The listing builds one solid part. Answer for the finished solid, in the listing's coordinates (mm). A direction names the side the tool comes from. Coordinates: 2 decimals unless noted, no trailing zeros. Order: outer loops, then holes, each group sorted by start corner. A loop starts at its lowest first (then second) coordinate and runs counter-clockwise, first axis right, second up. Notation, with made-up numbers: (85.5, -20) - (105.5, -20) arc R18 ccw to (105.5, -14) - close; hole circle Ø11 at (-18, 3). An arc over 180 degrees is marked (long way). One line per item, written item: value. Start each with the question number.
```python
from build123d import *

# Parameters (mm, degrees)
BOSS_EXTRUDE1_DEPTH = 6
SKETCH2_W           = 20
SKETCH2_H           = 30
BOSS_EXTRUDE2_DEPTH = 4
SKETCH3_W           = 20
SKETCH3_H           = 2
CUT_EXTRUDE1_DEPTH  = 6
SKETCH4_R           = 0.75
CUT_EXTRUDE2_DEPTH  = 172.161563774
SKETCH5_R           = 0.75
CUT_EXTRUDE3_DEPTH  = 153.773797585
SKETCH6_R           = 0.75
CUT_EXTRUDE4_DEPTH  = 174.032600725
SKETCH7_R           = 0.75
CUT_EXTRUDE5_DEPTH  = 191.462831696
FILLET1_R           = 4
SKETCH8_W           = 15
SKETCH8_H           = 30
BOSS_EXTRUDE3_DEPTH = 2
FILLET2_R           = 3
FILLET3_START       = 4.0000001
FILLET3_DEPTH       = 1.9999999
FILLET3_START_2     = 148.554137986
FILLET3_2_DEPTH     = 3.0000001
FILLET3_START_3     = 0.9999999
FILLET3_3_DEPTH     = 3.00000019
SKETCH9_R           = 0.75
CUT_EXTRUDE6_DEPTH  = 12
SKETCH10_R          = 1.1
CUT_EXTRUDE7_DEPTH  = 12
SKETCH11_R          = 1.1
CUT_EXTRUDE8_DEPTH  = 12
SKETCH12_R          = 0.75
CUT_EXTRUDE9_DEPTH  = 12
SKETCH13_R          = 2.1
CUT_EXTRUDE10_DEPTH = 6
SKETCH14_R          = 2.1
CUT_EXTRUDE11_DEPTH = 6


with BuildPart() as part:
    # Sketch1 → Boss-Extrude1 (new body)
    with BuildSketch(Plane.XY):
        Polygon((166.554138086, -30.981559499), (166.554138086, -0.981559499), (102.554138086, -0.981559499), (50.592613859, -30.981559499), (-9.407386141, -30.981559499), (-51.833793012, 11.444847372), (-101.833793012, 11.444847372), (-101.833793012, 7.444847372), (-53.490647262, 7.444847372), (-11.06424039, -34.981559499), (51.664410629, -34.981559499), (103.625934856, -4.981559499), (162.554138086, -4.981559499), (162.554138086, -30.981559499), align=None)
    extrude(amount=BOSS_EXTRUDE1_DEPTH)

    # Sketch2 → Boss-Extrude2 (add)
    with BuildSketch(Plane(origin=(166.554138086, 0, 0), x_dir=(0, 0, -1), z_dir=(1, 0, 0))):
        with Locations((10, -15.981559499)):
            Rectangle(SKETCH2_W, SKETCH2_H)
    extrude(amount=-BOSS_EXTRUDE2_DEPTH)

    # Sketch3 → Cut-Extrude1 (cut)
    with BuildSketch(Plane.XY.offset(6)):
        with Locations((-91.833793012, 8.444847372)):
            Rectangle(SKETCH3_W, SKETCH3_H)
    extrude(amount=-CUT_EXTRUDE1_DEPTH, mode=Mode.SUBTRACT)

    # Sketch4 → Cut-Extrude2 (cut, through all)
    with BuildSketch(Plane(origin=(0, -0.981559499, 0), x_dir=(1, 0, 0), z_dir=(0, 1, 0))):
        with Locations(Location((107.554138086, -3, 0), (0, 0, 180))):
            Circle(SKETCH4_R)
        with Locations(Location((117.554138086, -3, 0), (0, 0, 180))):
            Circle(SKETCH4_R)
        with Locations(Location((127.554138086, -3, 0), (0, 0, 180))):
            Circle(SKETCH4_R)
        with Locations(Location((137.554138086, -3, 0), (0, 0, 180))):
            Circle(SKETCH4_R)
        with Locations(Location((147.554138086, -3, 0), (0, 0, 180))):
            Circle(SKETCH4_R)
        with Locations(Location((157.554138086, -3, 0), (0, 0, 180))):
            Circle(SKETCH4_R)
    extrude(amount=-CUT_EXTRUDE2_DEPTH, mode=Mode.SUBTRACT)

    # Sketch5 → Cut-Extrude3 (cut, through all)
    with BuildSketch(Plane(origin=(26.063562252, -45.143414047, 0), x_dir=(0.8660254037844379, 0.5000000000000013, 0), z_dir=(-0.5000000000000013, 0.8660254037844379, 0))):
        with Locations(Location((33.323709096, -3, 0), (0, 0, 180))):
            Circle(SKETCH5_R)
        with Locations(Location((43.323709096, -3, 0), (0, 0, 180))):
            Circle(SKETCH5_R)
        with Locations(Location((53.323709096, -3, 0), (0, 0, 180))):
            Circle(SKETCH5_R)
        with Locations(Location((63.323709096, -3, 0), (0, 0, 180))):
            Circle(SKETCH5_R)
        with Locations(Location((73.323709096, -3, 0), (0, 0, 180))):
            Circle(SKETCH5_R)
        with Locations(Location((83.323709096, -3, 0), (0, 0, 180))):
            Circle(SKETCH5_R)
    extrude(amount=-CUT_EXTRUDE3_DEPTH, mode=Mode.SUBTRACT)

    # Sketch6 → Cut-Extrude4 (cut, through all)
    with BuildSketch(Plane(origin=(0, -30.981559499, 0), x_dir=(1, 0, 0), z_dir=(0, 1, 0))):
        with Locations(Location((45.592613859, -3, 0), (0, 0, 180))):
            Circle(SKETCH6_R)
        with Locations(Location((35.592613859, -3, 0), (0, 0, 180))):
            Circle(SKETCH6_R)
        with Locations(Location((25.592613859, -3, 0), (0, 0, 180))):
            Circle(SKETCH6_R)
        with Locations(Location((15.592613859, -3, 0), (0, 0, 180))):
            Circle(SKETCH6_R)
        with Locations(Location((5.592613859, -3, 0), (0, 0, 180))):
            Circle(SKETCH6_R)
        with Locations(Location((-4.407386141, -3, 0), (0, 0, 180))):
            Circle(SKETCH6_R)
    extrude(amount=-CUT_EXTRUDE4_DEPTH, mode=Mode.SUBTRACT)

    # Sketch7 → Cut-Extrude5 (cut, through all)
    with BuildSketch(Plane(origin=(-20.19447282, -20.19447282, 0), x_dir=(0, 0, -1), z_dir=(0.7071067811865487, 0.7071067811865464, 0))):
        with Locations(Location((-3, -10.25524428, 0), (0, 0, 90))):
            Circle(SKETCH7_R)
        with Locations(Location((-3, -0.25524428, 0), (0, 0, 90))):
            Circle(SKETCH7_R)
        with Locations(Location((-3, 9.74475572, 0), (0, 0, 90))):
            Circle(SKETCH7_R)
        with Locations(Location((-3, 19.74475572, 0), (0, 0, 90))):
            Circle(SKETCH7_R)
        with Locations(Location((-3, 29.74475572, 0), (0, 0, 90))):
            Circle(SKETCH7_R)
        with Locations(Location((-3, 39.74475572, 0), (0, 0, 90))):
            Circle(SKETCH7_R)
    extrude(amount=-CUT_EXTRUDE5_DEPTH, mode=Mode.SUBTRACT)

    # Fillet1
    fillet1_edges = [part.edges().sort_by_distance(p)[0] for p in [
        (162.554138086, -4.981559499, 3),
        (162.554138086, -2.981559499, 0),
    ]]
    fillet(fillet1_edges, radius=FILLET1_R)

    # Sketch8 → Boss-Extrude3 (add)
    with BuildSketch(Plane.XY.offset(6)):
        with Locations((159.054138086, -15.981559499)):
            Rectangle(SKETCH8_W, SKETCH8_H)
    extrude(amount=-BOSS_EXTRUDE3_DEPTH)

    # Fillet2
    # the kernel refuses this fillet: 3 mm, written as the material it adds along each edge
    with BuildSketch(Plane(origin=(158.554138086, -8.981559499, 4), x_dir=(1, 0, 0), z_dir=(0, -1, 0))) as fillet2_piece_1:
        with BuildLine():
            CenterArc((4 - FILLET2_R, -FILLET2_R), FILLET2_R, 0, 90)
            Line((4, -FILLET2_R), (4, 0))
            Line((4, 0), (4 - FILLET2_R, 0))
        make_face()
    revolve(axis=Axis((158.554138086, -8.981559499, 4), (0, 0, 1)), revolution_arc=90)
    with BuildSketch(Plane(origin=(151.554138086, -4.981559499, 4), x_dir=(0, -1, 0), z_dir=(1, 0, 0))) as fillet2_piece_2_section:
        with BuildLine():
            CenterArc((FILLET2_R, FILLET2_R), FILLET2_R, 180, 90)
            Line((0, FILLET2_R), (0, 0))
            Line((0, 0), (FILLET2_R, 0))
        make_face()
    fillet2_piece_2 = extrude(amount=7, mode=Mode.PRIVATE)
    fillet2_piece_2 = fillet2_piece_2 - Plane(origin=(157.554138086, -4.981559499, 3), x_dir=(-1, 0, 0), z_dir=(0, 1, 0)) * Cylinder(0.75, 27, mode=Mode.PRIVATE)
    add(fillet2_piece_2)
    with BuildSketch(Plane(origin=(162.554138086, -8.981559499, 4), x_dir=(0, 0, -1), z_dir=(0, -1, 0))) as fillet2_piece_3:
        with BuildLine():
            CenterArc((FILLET2_R, -FILLET2_R), FILLET2_R, 90, 90)
            Line((0, -FILLET2_R), (0, 0))
            Line((0, 0), (FILLET2_R, 0))
        make_face()
    extrude(amount=22)

    # Fillet3: read off the stored shape, not the designer's step
    # Fillet3 outline → Fillet3 (add)
    with BuildSketch(Plane.XY.offset(FILLET3_START)):
        with BuildLine():
            ThreePointArc((148.554138086, -4.981559499), (150.67545843, -5.860239155), (151.554138086, -7.981559499))
            Line((151.554138086, -7.981559499), (151.554138086, -4.981559499))
            Line((151.554138086, -4.981559499), (148.554138086, -4.981559499))
        make_face()
    extrude(amount=FILLET3_DEPTH)

    # Fillet3 2 outline → Fillet3 2 (add)
    with BuildSketch(Plane.YZ.offset(FILLET3_START_2)):
        with BuildLine():
            Line((-4.981559499, 4.0000001), (-7.981559499, 4))
            ThreePointArc((-7.981559499, 4), (-5.860239155, 3.121320344), (-4.981559499, 1))
            Line((-4.981559499, 1), (-4.981559499, 4.0000001))
        make_face()
    extrude(amount=FILLET3_2_DEPTH)

    # Fillet3 3 outline → Fillet3 3 (cut)
    with BuildSketch(Plane.XY.offset(FILLET3_START_3)):
        with BuildLine():
            Line((151.554138085, -9), (151.554138086, -7.981559499))
            ThreePointArc((151.554138086, -7.981559499), (150.67545843, -5.860239155), (148.554138086, -4.981559499))
            Line((148.554138086, -4.981559499), (148.554137986, -9))
            Line((148.554137986, -9), (151.554138085, -9))
        make_face()
    extrude(amount=FILLET3_3_DEPTH, mode=Mode.SUBTRACT)

    # Sketch9 → Cut-Extrude6 (cut)
    with BuildSketch(Plane(origin=(0, 11.444847372, 0), x_dir=(1, 0, 0), z_dir=(0, 1, 0))):
        with Locations(Location((-56.833793012, -3, 0), (0, 0, 180))):
            Circle(SKETCH9_R)
        with Locations(Location((-66.833793012, -3, 0), (0, 0, 180))):
            Circle(SKETCH9_R)
        with Locations(Location((-76.833793012, -3, 0), (0, 0, 180))):
            Circle(SKETCH9_R)
    extrude(amount=-CUT_EXTRUDE6_DEPTH, mode=Mode.SUBTRACT)

    # Sketch10 → Cut-Extrude7 (cut)
    with BuildSketch(Plane.XZ.offset(-9.444847372)):
        with Locations(Location((-98.833793012, 3, 0), (0, 0, 270))):
            Circle(SKETCH10_R)
    extrude(amount=-CUT_EXTRUDE7_DEPTH, mode=Mode.SUBTRACT)

    # Sketch11 → Cut-Extrude8 (cut)
    with BuildSketch(Plane.XZ.offset(-9.444847372)):
        with Locations(Location((-86.833793012, 3, 0), (0, 0, 270))):
            Circle(SKETCH11_R)
    extrude(amount=-CUT_EXTRUDE8_DEPTH, mode=Mode.SUBTRACT)

    # Sketch12 → Cut-Extrude9 (cut)
    with BuildSketch(Plane.XZ.offset(-9.444847372)):
        with Locations(Location((-92.833793012, 3, 0), (0, 0, 270))):
            Circle(SKETCH12_R)
    extrude(amount=-CUT_EXTRUDE9_DEPTH, mode=Mode.SUBTRACT)

    # Sketch13 → Cut-Extrude10 (cut)
    with BuildSketch(Plane(origin=(166.554138086, 0, 0), x_dir=(0, 0, -1), z_dir=(1, 0, 0))):
        with Locations(Location((1, -20.981559499, 0), (0, 0, 90))):
            Circle(SKETCH13_R)
    extrude(amount=-CUT_EXTRUDE10_DEPTH, mode=Mode.SUBTRACT)

    # Sketch14 → Cut-Extrude11 (cut)
    with BuildSketch(Plane(origin=(166.554138086, 0, 0), x_dir=(0, 0, -1), z_dir=(1, 0, 0))):
        with Locations(Location((13, -20.981559499, 0), (0, 0, 90))):
            Circle(SKETCH14_R)
    extrude(amount=-CUT_EXTRUDE11_DEPTH, mode=Mode.SUBTRACT)


solid = part.part
```
(1) For faces 4 (the face through (21, -30.982, 3)), 5 (the face through (-68, 7.445, 3)), 6 (the face through (155, -19, 4)), 7 (the face through (77.281, -20.192, 2.958)), determine the directions among +Z, -Z, +X, -X, +Y, -Y from which every point of the face is accessible in a straight line to the end or side of a thin tool.
(2) Flat-ended cylindrical pins translate along their axes: pin 1 Ø3.5 at (y, z) = (-20.98, -1) entering from +X; pin 2 Ø1.6 at (y, z) = (8, 3) entering from -X; pin 3 Ø8 at (y, z) = (-26, -4.5) entering from -X. Find the tip coordinate at first contact, or state that the pin passes through.
(3) The part is cut by section A-A on x = 42.5. Determine the outline of the cut face in (y, z), plus the area to 3 significant figures.
(4) The part is cut by section B-B on x = 78. Determine the outline of the cut face in (y, z), plus the area to 3 significant figures.
(5) Consider probe 1 along Y at (x, z) = (164.05, -1); probe 2 along Z at (x, y) = (-69, 8); probe 3 along X at (y, z) = (-10.5, -10.5). Determine where each line is inside the solid, lowest interval first.
(6) For a pull along X with two mould halves and no side action, classify faces 1 (the face through (125, -4.982, 3)), 2 (the face through (166.554, -16, -7)), 3 (the face through (-92, 9.445, 4)) as pulls with the +X half, pulls with the -X half, needs draft (parallel to the pull), parting line crosses it, or undercut.
Completed:
1. face 4: +Z, -Z, +Y
1. face 5: +Z, -Z, -X, -Y
1. face 6: -Z, -Y
1. face 7: +Z, -Z, -Y
2. pin 1: stops at x = 78.4
2. pin 2: stops at x = -81.83
2. pin 3: stops at x = 162.55
3. outline: (-34.98, 0) - (-30.98, 0) - (-30.98, 6) - (-34.98, 6) - close
3. area: 24.0 mm2
4. outline: (-19.78, 0) - (-15.16, 0) - (-15.16, 6) - (-19.78, 6) - close
4. area: 27.7 mm2
5. probe 1: y = -30.98 to -23.08, -18.88 to -0.98
5. probe 2: z = 0 to 6
5. probe 3: x = 162.55 to 166.55
6. face 1: undercut
6. face 2: pulls with the +X half
6. face 3: needs draft
